Check sheet for the modelled part. Datum: model origin and axes. Units: mm. A direction names the side the tool comes from. Give positions to 0.01 mm unless a question says otherwise; leave off trailing zeros. Order: outer loops, then holes, each group sorted by start corner. A loop starts at its lowest first (then second) coordinate and runs counter-clockwise, first axis right, second up. Notation, with made-up numbers: M -22.75,39.5 L 25.25,39.5 A16 ccw 25.25,44.5 Z; hole C -28,48.5 d11. An arc over 180 degrees is marked long. Return JSON: item names as keys, results as strings. Group by question number.
from build123d import *

# Parameters (mm, degrees)
SKETCH_R        = 1.6
PAD_DEPTH       = 26.7
SKETCH001_W     = 56.65
SKETCH001_H     = 70.73
SKETCH001_W_2   = 31.75
SKETCH001_H_2   = 28
POCKET_DEPTH    = 24.2
SKETCH002_W     = 36.75
SKETCH002_H     = 30.5
POCKET001_DEPTH = 15.2
SKETCH003_W     = 12.43
SKETCH003_H     = 2.95
SKETCH003_W_2   = 9.39
POCKET002_DEPTH = 20.2
SKETCH004_R     = 14.5
POCKET003_DEPTH = 17.25
SKETCH005_R     = 3.5
POCKET004_DEPTH = 2.5
FILLET_R        = 1
FILLET001_R     = 1


with BuildPart() as part:
    # Sketch → Pad (new body)
    with BuildSketch(Plane.XY):
        Polygon((-30.825, -68.49), (30.825, -68.49), (30.825, 7.49), (18.375, 7.49), (18.375, 37.99), (-18.375, 37.99), (-18.375, 7.49), (-30.825, 7.49), align=None)
        with Locations((-25.25, 0)):
            Circle(SKETCH_R, mode=Mode.SUBTRACT)
        with Locations((25.25, 0)):
            Circle(SKETCH_R, mode=Mode.SUBTRACT)
        Polygon((26.88, -51.57), (25.505, -49.18843), (22.755, -49.18843), (21.38, -51.57), (22.755, -53.95157), (25.505, -53.95157), align=None, mode=Mode.SUBTRACT)
        Polygon((-6.14, 0.5), (-7.515, 2.88157), (-10.265, 2.88157), (-11.64, 0.5), (-10.265, -1.88157), (-7.515, -1.88157), align=None, mode=Mode.SUBTRACT)
        Polygon((20.425, -1.88157), (21.8, 0.5), (20.425, 2.88157), (17.675, 2.88157), (16.3, 0.5), (17.675, -1.88157), align=None, mode=Mode.SUBTRACT)
        Polygon((-22.755, -52.68157), (-21.38, -50.3), (-22.755, -47.91843), (-25.505, -47.91843), (-26.88, -50.3), (-25.505, -52.68157), align=None, mode=Mode.SUBTRACT)
    extrude(amount=PAD_DEPTH)

    # Sketch001 (on Face36 of Pad) → Pocket (cut)
    with BuildSketch(Plane.XY.offset(26.7)):
        with Locations((0, -30.375)):
            Rectangle(SKETCH001_W, SKETCH001_H)
        with Locations((0, 21.49)):
            Rectangle(SKETCH001_W_2, SKETCH001_H_2)
    extrude(amount=-POCKET_DEPTH, mode=Mode.SUBTRACT)

    # Sketch002 (on Face5 of Pocket) → Pocket001 (cut)
    with BuildSketch(Plane.XY.offset(26.7)):
        with Locations((0, 22.74)):
            Rectangle(SKETCH002_W, SKETCH002_H)
    extrude(amount=-POCKET001_DEPTH, mode=Mode.SUBTRACT)

    # Sketch003 (on Face5 of Pocket001) → Pocket002 (cut)
    with BuildSketch(Plane.XY.offset(26.7)):
        with Locations((-11.43, -67.015)):
            Rectangle(SKETCH003_W, SKETCH003_H)
        with Locations((18.8, -67.015)):
            Rectangle(SKETCH003_W_2, SKETCH003_H)
    extrude(amount=-POCKET002_DEPTH, mode=Mode.SUBTRACT)

    # Sketch004 (on Face1 of Pocket002) → Pocket003 (cut)
    with BuildSketch(Plane.XZ.offset(68.49)):
        with Locations((0, -9.5)):
            Circle(SKETCH004_R)
    extrude(amount=-POCKET003_DEPTH, mode=Mode.SUBTRACT)

    # Sketch005 (on Face46 of Pocket003) → Pocket004 (cut)
    with BuildSketch(Plane.XY.offset(2.5)):
        with Locations((25.25, -22)):
            Circle(SKETCH005_R)
        with Locations((-25.25, -22)):
            Circle(SKETCH005_R)
    extrude(amount=-POCKET004_DEPTH, mode=Mode.SUBTRACT)

    # Fillet
    fillet_edges = [part.edges().sort_by_distance(p)[0] for p in [
        (15.875, 21.49, 11.5),
        (0, 35.49, 11.5),
        (-15.875, 21.49, 11.5),
        (-17.645, -67.115, 26.7),
        (-5.215, -67.115, 26.7),
        (14.105, -67.115, 26.7),
        (23.495, -67.115, 26.7),
    ]]
    fillet(fillet_edges, radius=FILLET_R)

    # Fillet001
    fillet001_edges = [part.edges().sort_by_distance(p)[0] for p in [
        (-28.325, -30.375, 26.7),
        (-23.485, -65.74, 26.7),
        (4.445, -65.74, 26.7),
        (28.325, -30.375, 26.7),
        (26.41, -65.74, 26.7),
        (0, 4.99, 26.7),
    ]]
    fillet(fillet001_edges, radius=FILLET001_R)


solid = part.part
1) Depth check by flat-ended pin: P1, Ø14, axis at x = 6, y = 27, coming from the +Z side; P2, Ø1.5, axis at x = 21.5, z = 2.5, coming from the +Y side; P3, Ø3, axis at x = -8, y = -67, coming from the +Z side. Enter the tip coordinate at first touch or a pass-through.
2) Material ranges on line 1 along Y through (x, z) = (25.25, 1.15); line 2 along X through (y, z) = (-22, 1.9) (3 decimals); line 3 along Y through (x, z) = (8.5, 9), recorded low to high.
3) Release check for a two-part mould opening along X. For faces 1 (the face through (-22.08, -51.51, 1.23)), 2 (the face through (-0.1, 6.3, 26.7)), 3 (the face through (-18.375, 23, 6)) record: released by +X, released by -X, zero draft, split by the parting line, or undercut.
4) Tool access check on faces 4 (the face through (0, 22, 2.5)), 5 (the face through (-24, -52.682, 1)), 6 (the face through (27.13, -19.05, 1.27)). Record the directions out of +Z, -Z, +X, -X, +Y, -Y that give a thin tool (end or side, any length) a straight path to the whole face; none if there is none.
5) Sectioned sample at A-A on z = 21.75. Record the boundary of the cut face in (x, y) (3 decimals), then the cut area to 3 significant figures.
6) Sectioned sample at B-B on y = -22. Record the boundary of the cut face in (x, z) (3 decimals).
Reply:
{
 "1": {"P1": "z = 2.5", "P2": "y = 7.49", "P3": "z = 6.5"},
 "2": {"line 1": "-68.49 to -53.95, -49.19 to -25.5, -18.5 to -1.6, 1.6 to 7.49", "line 2": "-30.825 to -28.75, -21.75 to 21.75, 28.75 to 30.825", "line 3": "-68.49 to -65.74, 4.99 to 7.49, 35.49 to 37.99"},
 "3": {"face 1": "undercut", "face 2": "zero draft", "face 3": "released by -X"},
 "4": {"face 4": "+Z", "face 5": "+Z, -Z", "face 6": "-Z"},
 "5": {"outline": "M -30.825,-68.49 L -17.645,-68.49 L -17.645,-66.74 A1 ccw -18.645,-65.74 L -28.325,-65.74 L -28.325,4.99 L 28.325,4.99 L 28.325,-65.74 L 24.495,-65.74 A1 ccw 23.495,-66.74 L 23.495,-68.49 L 30.825,-68.49 L 30.825,7.49 L -30.825,7.49 Z; M -5.215,-68.49 L 14.105,-68.49 L 14.105,-66.74 A1 ccw 13.105,-65.74 L -4.215,-65.74 A1 ccw -5.215,-66.74 Z", "area": "616 mm^2"},
 "6": {"outline": "M -30.825,0 L -28.75,0 L -28.75,2.5 L -28.325,2.5 L -28.325,25.7 A1 ccw -29.325,26.7 L -30.825,26.7 Z; M -21.75,0 L 21.75,0 L 21.75,2.5 L -21.75,2.5 Z; M 28.325,2.5 L 28.75,2.5 L 28.75,0 L 30.825,0 L 30.825,26.7 L 29.325,26.7 A1 ccw 28.325,25.7 Z"}
}
